from build123d import *

# Parameters (mm, degrees)
ESQUISSE1_W                  = 6
ESQUISSE1_H                  = 20
CHANFREIN1_SIZE              = 0.5
R_P_TITION_CIRCULAIRE1_COUNT = 4
TROU_TARAUD_M12X1_752_D      = 10.2


with BuildPart() as part:
    # Esquisse1 → Base-Révolution (revolve)
    with BuildSketch(Plane.XY, mode=Mode.PRIVATE) as base_r_volution_sk:
        with Locations((3, 10)):
            Rectangle(ESQUISSE1_W, ESQUISSE1_H)
    revolve(base_r_volution_sk.sketch.rotate(Axis((-6.22145749, 0, 0), (1, 0, 0)), 90), axis=Axis((-6.22145749, 0, 0), (1, 0, 0)))

    # Chanfrein1
    chanfrein1_edges = [part.edges().sort_by_distance(p)[0] for p in [
        (6, 0, -20),
        (0, 0, -20),
    ]]
    chamfer(chanfrein1_edges, length=CHANFREIN1_SIZE)

    # Esquisse2 → Trou radial (revolve, cut)
    with BuildSketch(Plane.XY, mode=Mode.PRIVATE) as trou_radial_sk:
        Polygon((5, 20), (3, 20), (3, 13.798278762), (5, 15), align=None)
    trou_radial = revolve(trou_radial_sk.sketch.rotate(Axis((3, 20, 0), (0, -1, 0)), 180), axis=Axis((3, 20, 0), (0, -1, 0)), mode=Mode.SUBTRACT)

    # Répétition circulaire1: Trou radial ×4 about axis
    r_p_tition_circulaire1_axis = Axis((43.77854251, 0, 0), (-1, 0, 0))
    for i in range(1, R_P_TITION_CIRCULAIRE1_COUNT):
        add(trou_radial.rotate(r_p_tition_circulaire1_axis, i * 360 / R_P_TITION_CIRCULAIRE1_COUNT), mode=Mode.SUBTRACT)

    # Trou taraudé M12x1.752 (through all)
    with Locations(Plane(origin=(6, 0, 0), x_dir=(0, 0, -1), z_dir=(1, 0, 0))):
        with Locations((0, 0)):
            Hole(TROU_TARAUD_M12X1_752_D / 2)


solid = part.part
Check sheet for the modelled part. Datum: model origin and axes. Units: mm. A direction names the side the tool comes from. Give positions to 0.01 mm unless a question says otherwise; leave off trailing zeros. Use a Markdown table: item, result. Add a question column.
Q1. Mould release check, pull along Y, two halves, no side actions. Record for faces 6 (the conical face through (3.35, -14.01, 0.02)), 7 (the cylindrical face through (3.035, -6.007, 19.076)), 8 (the flat face through (0, 4, -4)), 9 (the conical face through (3.35, -0.02, -14.01)): pulls with the +Y half, pulls with the -Y half, needs draft (parallel to the pull), parting line crosses it, or undercut.
Q2. Scan lines: line 1 along X through (y, z) = (0, 17.1); line 2 along Y through (x, z) = (3.9, 3.5); line 3 along Z through (x, y) = (3.4, 16). Record each from-to range of solid material in increasing order. Write a range as [from, to].
Q3. Tool access check on faces 1 (the cylindrical face through (3, -4.5, 2.4)), 2 (the cylindrical face through (4.6, 17.5, 1.2)), 3 (the cylindrical face through (4.474, -17.535, 1.352)), 4 (the cylindrical face through (3, 2, 18)), 5 (the cylindrical face through (1.092, -0.601, -17.535)). Record the directions out of +Z, -Z, +X, -X, +Y, -Y that give a thin tool (end or side, any length) a straight path to the whole face; none if there is none.
Q4. Go/stop test with flat-tipped pins: pin 1 (1 mm diameter, centred on x = 3, z = 3, fed in from -Y); pin 2 (1 mm diameter, centred on x = 3.5, z = -2, fed in from -Y); pin 3 (1.5 mm diameter, centred on y = -3.5, z = 16, fed in from -X). Record where each tip stops, or that it passes through.
Verdict:
| question | item | result |
|---|---|---|
| 1 | face 6 | pulls with the -Y half |
| 1 | face 7 | parting line crosses it |
| 1 | face 8 | needs draft |
| 1 | face 9 | undercut |
| 2 | line 1 | [0, 1], [5, 6] |
| 2 | line 2 | [-19.69, -3.71], [3.71, 19.69] |
| 2 | line 3 | [-12, -1.96], [1.96, 12] |
| 3 | face 1 | +X, -X |
| 3 | face 2 | +Y |
| 3 | face 3 | -Y |
| 3 | face 4 | +Z |
| 3 | face 5 | -Z |
| 4 | pin 1 | y = -19.84 |
| 4 | pin 2 | y = -19.92 |
| 4 | pin 3 | x = 0 |
